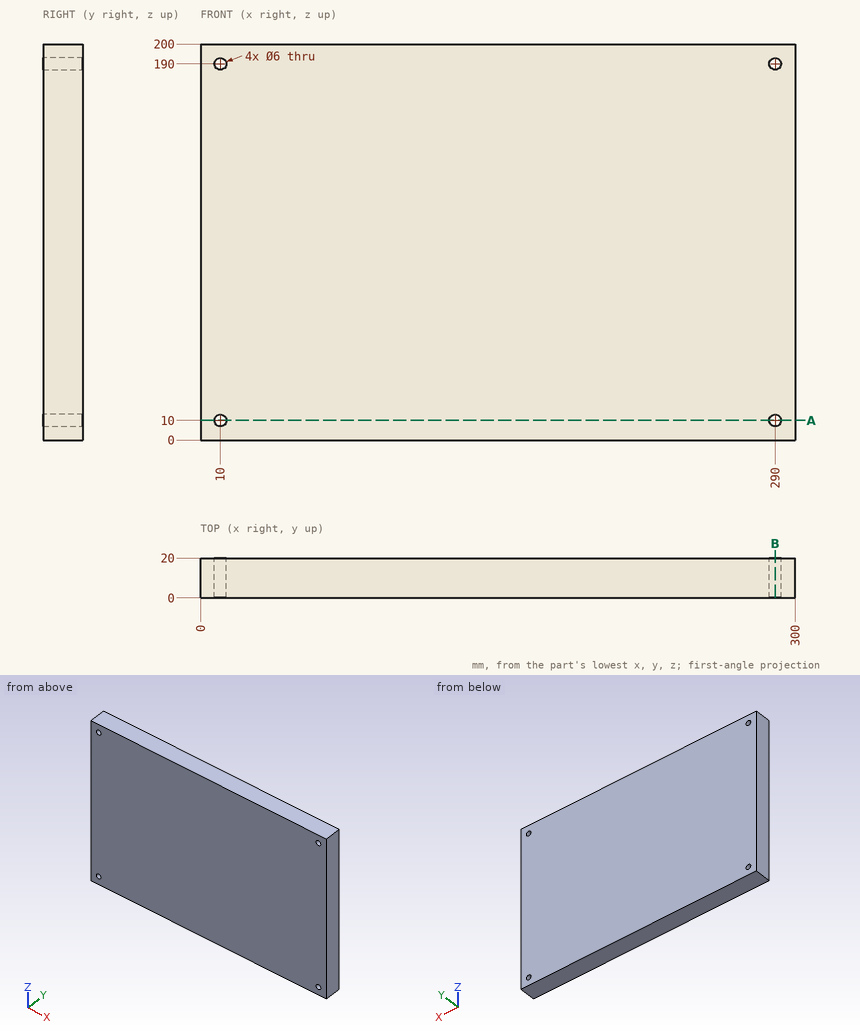
Verification items for this drawing (mm, ordinates from the low corner). Give positions to 0.01 mm unless a question says otherwise; leave off trailing zeros. Order: outer loops, then holes, each group sorted by start corner. A loop starts at its lowest first (then second) coordinate and runs counter-clockwise, first axis right, second up.
1) Material ranges on probe 1 along Z at (x, y) = (290, 11.75); probe 2 along X at (y, z) = (14, 10), recorded low to high.
Results are:
probe 1: z = 0 to 7, 13 to 187, 193 to 200
probe 2: x = 0 to 7, 13 to 287, 293 to 300
2) Cross-section at B-B (x = 290). Record the boundary of the cut face in (y, z).
Results are:
outline: (0, 0) - (20, 0) - (20, 7) - (0, 7) - close; (0, 13) - (20, 13) - (20, 187) - (0, 187) - close; (0, 193) - (20, 193) - (20, 200) - (0, 200) - close
3) Cross-section at A-A (z = 10). Record the boundary of the cut face in (x, y), then the cut area to 3 significant figures.
Results are:
outline: (0, 0) - (7, 0) - (7, 20) - (0, 20) - close; (13, 0) - (287, 0) - (287, 20) - (13, 20) - close; (293, 0) - (300, 0) - (300, 20) - (293, 20) - close
area: 5,760 mm2
